from build123d import *

# Parameters (mm, degrees)
F0_W     = 16
F0_H     = 12
F1_DEPTH = 16
F2_T     = -1
F4_D     = 4
F5_DEPTH = 5
F6_R     = 1


with BuildPart() as f1:
    # F0 (on Top) → F1 (new body)
    with BuildSketch(Plane.XY):
        Rectangle(F0_W, F0_H)
    extrude(amount=F1_DEPTH)

    # F2
    f2_openings = [f1.faces().sort_by_distance(p)[0] for p in [
        (0, 0, 16),
    ]]
    offset(amount=F2_T, openings=f2_openings)

    # F4 (through all)
    with Locations(Plane.XZ.offset(6)):
        with Locations((0, 8)):
            Hole(F4_D / 2)

    # F5 (add): a face of the model
    f5_faces = [f1.faces().sort_by_distance(p)[0] for p in [
        (0, 0, 0),
    ]]
    extrude(f5_faces, amount=F5_DEPTH)

    # F6
    f6_edges = [f1.edges().sort_by_distance(p)[0] for p in [
        (8, -6, 5.5),
        (-8, -6, 5.5),
        (8, 6, 5.5),
        (-8, 6, 5.5),
    ]]
    fillet(f6_edges, radius=F6_R)


solid = f1.part
Part model, mm, in its own coordinate system. A direction names the side the tool comes from. Give positions to 0.01 mm unless a question says otherwise; leave off trailing zeros. Loops run counter-clockwise (first coordinate to the right, second up) from the corner with the lowest first, then second, coordinate; pieces in that order, holes last. Notation, with made-up numbers: M -14.5,40 L 8.5,40 A22 cw 8.5,74 Z; hole C 38.5,-31 d4. An arc over 180 degrees is marked long. Put each result on its own line as item: value. Start each with the question number.
1) Saw through at D-D (y = 4). List the corners of the cut face in (x, z).
2) Pull direction Z, two halves, no side cores. Call faces 1 (the flat face through (0, 0, -5)), 2 (the flat face through (-0.1, -6, 5.6)), 3 (the flat face through (0, 5.4, 16)), 4 (the cylindrical face through (0.26, 5.507, 9.983)): +Z half, -Z half, draft (parallel to the pull), parting line (faces both ways), or undercut.
3) Flat gauge pins, fed straight in: pin 1 (5 mm diameter, centred on x = -2.5, y = -1, fed in from +Z); pin 2 (2.5 mm diameter, centred on x = 0, z = 8, fed in from -Y). Where does each tip first touch, or does it go through?
4) 3-axis set-ups, long thin cutter, end or side, ignore diameter. For faces 5 (the flat face through (0, 0, 1)), 6 (the flat face through (-8, 0, 6)): which of +Z, -Z, +X, -X, +Y, -Y reach the whole face in a straight line?
5) Saw through at B-B (x = 0). List the corners of the cut face in (y, z).
6) Saw through at A-A (z = 8). List the corners of the cut face in (x, y).
7) Probe probe 1 along Y at (x, z) = (4.5, 12.25); probe 2 along X at (y, z) = (2.75, 14.25); probe 3 along Z at (x, y) = (0, 5.65). List the from-to ranges inside material, lowest first.
8) Saw through at C-C (z = 13.25). List the corners of the cut face in (x, y).
Numbers:
1. outline: M -8,-5 L 8,-5 L 8,16 L 7,16 L 7,1 L -7,1 L -7,16 L -8,16 Z
2. face 1: -Z half
2. face 2: draft
2. face 3: +Z half
2. face 4: undercut
3. pin 1: z = 1
3. pin 2: through
4. face 5: +Z
4. face 6: +Z, -Z, -X, +Y, -Y
5. outline: M -6,-5 L 6,-5 L 6,6 L 5,6 L 5,1 L -5,1 L -5,6 L -6,6 Z; M -6,10 L -5,10 L -5,16 L -6,16 Z; M 5,10 L 6,10 L 6,16 L 5,16 Z
6. outline: M -8,-5 A1 ccw -7,-6 L -2,-6 L -2,-5 L -7,-5 L -7,5 L -2,5 L -2,6 L -7,6 A1 ccw -8,5 Z; M 2,-6 L 7,-6 A1 ccw 8,-5 L 8,5 A1 ccw 7,6 L 2,6 L 2,5 L 7,5 L 7,-5 L 2,-5 Z
7. probe 1: -6 to -5, 5 to 6
7. probe 2: -8 to -7, 7 to 8
7. probe 3: -5 to 6, 10 to 16
8. outline: M -8,-5 A1 ccw -7,-6 L 7,-6 A1 ccw 8,-5 L 8,5 A1 ccw 7,6 L -7,6 A1 ccw -8,5 Z; hole M -7,-5 L 7,-5 L 7,5 L -7,5 Z
